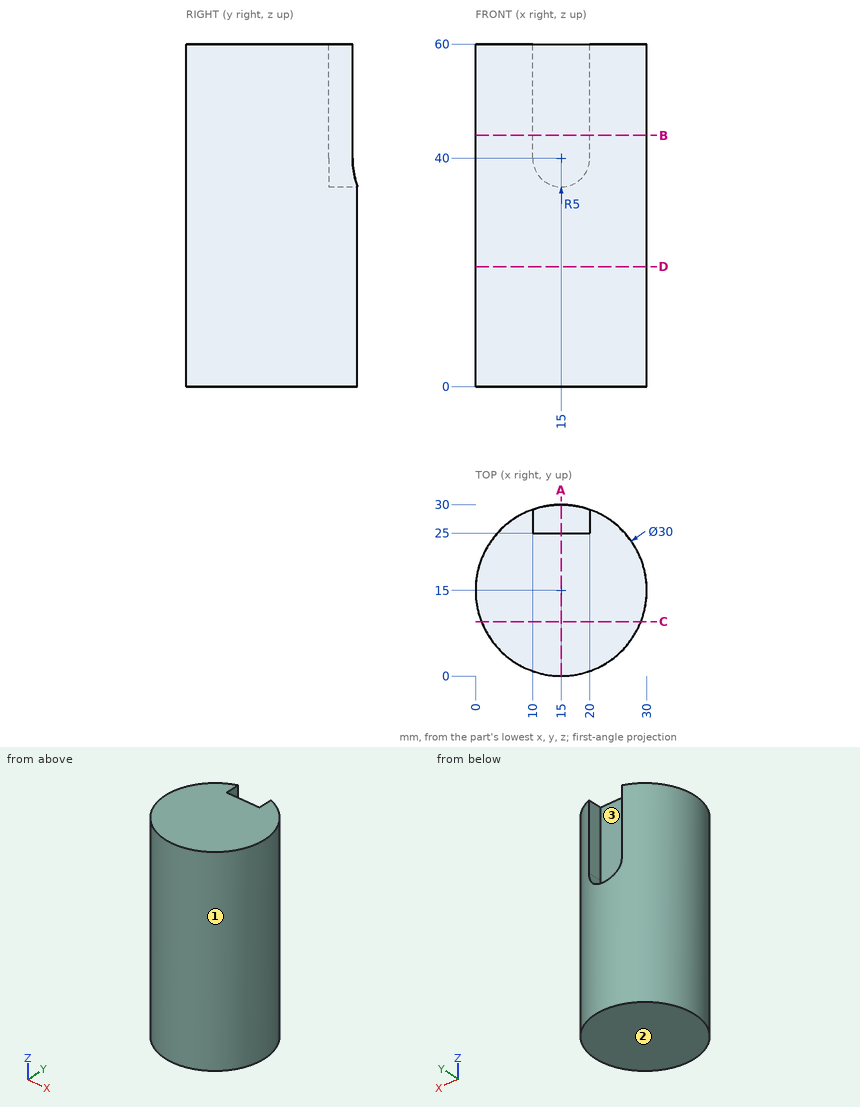
Can you work these out from the drawing? Everything is in mm from the part's minimum corner. Coordinates: 2 decimals unless noted, no trailing zeros. Loops run counter-clockwise (first coordinate to the right, second up) from the corner with the lowest first, then second, coordinate; pieces in that order, holes last.
1) Imagine slicing it at B-B on z = 44. List the corners of the cut face in (x, y) for me, plus the area to 3 significant figures.
2) For pin 1 (3.5 mm diameter, centred on y = 26, z = 50.5, fed in from +X); pin 2 (3 mm diameter, centred on x = 10.5, z = 36, fed in from +Y); pin 3 (4.5 mm diameter, centred on y = 27.5, z = 49.5, fed in from -X), each with a flat end and sliding along its axis, tell me the tip position at first contact or that it passes through.
3) Imagine slicing it at C-C on y = 9.5. List the corners of the cut face in (x, z) for me, plus the area to 3 significant figures.
4) Imagine slicing it at A-A on x = 15. List the corners of the cut face in (y, z) for me, plus the area to 4 significant figures.
5) Imagine slicing it at D-D on z = 21. List the corners of the cut face in (x, y) for me, plus the area to 3 significant figures.
6) I need wall thicknesses on probe 1 along Y at (x, z) = (28, 4); probe 2 along Y at (x, z) = (23, 16); probe 3 along X at (y, z) = (24.5, 15). Which ranges of each line are inside material? Lowest first, please.
7) Thinking about a two-plate mould opening in X: for the marked faces 1, 2 and 3, which applies, pulls with the +X half, pulls with the -X half, needs draft (parallel to the pull), parting line crosses it, or undercut?
Completed:
1. outline: (10, 25) - (10, 29.14) arc R15 ccw (long way) to (20, 29.14) - (20, 25) - close
1. area: 660 mm2
2. pin 1: stops at x = 26.81
2. pin 2: stops at y = 29.7
2. pin 3: stops at x = 4.05
3. outline: (1.04, 0) - (28.96, 0) - (28.96, 60) - (1.04, 60) - close
3. area: 1,670 mm2
4. outline: (0, 0) - (30, 0) - (30, 35) - (25, 35) - (25, 60) - (0, 60) - close
4. area: 1,675 mm2
5. outline: circle Ø30 at (15, 15)
5. area: 707 mm2
6. probe 1: y = 7.52 to 22.48
6. probe 2: y = 2.31 to 27.69
6. probe 3: x = 3.39 to 26.61
7. face 1: parting line crosses it
7. face 2: needs draft
7. face 3: undercut
